```python
from build123d import *

# Parameters (mm, degrees)
SKETCH_1_W               = 40
SKETCH_1_H               = 24
EXTRUDE_1_DEPTH          = 20
EXTRUDE_2_DEPTH          = 1
EXTRUDE_2_2_DEPTH        = 1
EXTRUDE_2_3_DEPTH        = 1
EXTRUDE_2_4_DEPTH        = 1
SKETCH_1_6_W             = 1
SKETCH_1_6_H             = 24
EXTRUDE_4_DEPTH          = 20
SKETCH_2_R               = 4
EXTRUDE_5_DEPTH          = 2
FILLET_1_R               = 2
CHAMFER_1_SIZE           = 1
CHAMFER_2_SIZE           = 1
SKETCH_3_R               = 1
EXTRUDE_6_DEPTH          = 5
MIRROR_4_COPY_1_SKETCH_R = 1
MIRROR_4_COPY_1_DEPTH    = 5
MIRROR_4_COPY_2_SKETCH_R = 1
MIRROR_4_COPY_2_DEPTH    = 5


with BuildPart() as part:
    # Sketch 1 → Extrude 1 (new body)
    with BuildSketch(Plane(origin=(0, 0, 0), x_dir=(1, 0, 0), z_dir=(0, 1, 0))):
        Rectangle(SKETCH_1_W, SKETCH_1_H)
    extrude(amount=EXTRUDE_1_DEPTH)



with BuildPart() as body_2:
    # Sketch 1_4 → Extrude 2 (new body)
    with BuildSketch(Plane(origin=(0, 0, 0), x_dir=(1, 0, 0), z_dir=(0, 1, 0))):
        with BuildLine():
            Line((-21, 0), (-21, 9))
            Line((-21, 9), (-29, 6))
            Line((-29, 6), (-29, 2.5))
            Line((-29, 2.5), (-23, 2))
            ThreePointArc((-23, 2), (-21.585786438, 1.414213562), (-21, 0))
        make_face()
    extrude(amount=EXTRUDE_2_DEPTH)


with BuildPart() as body_3:
    # Sketch 1_4 → Extrude 2 2 (new body)
    with BuildSketch(Plane(origin=(0, 0, 0), x_dir=(1, 0, 0), z_dir=(0, 1, 0))):
        with BuildLine():
            Line((-29, -6), (-21, -9))
            Line((-21, -9), (-21, 0))
            ThreePointArc((-21, 0), (-21.585786438, -1.414213562), (-23, -2))
            Line((-23, -2), (-29, -2.5))
            Line((-29, -2.5), (-29, -6))
        make_face()
    extrude(amount=EXTRUDE_2_2_DEPTH)


with BuildPart() as body_4:
    # Sketch 1_4 → Extrude 2 3 (new body)
    with BuildSketch(Plane(origin=(0, 0, 0), x_dir=(1, 0, 0), z_dir=(0, 1, 0))):
        with BuildLine():
            Line((29, 6), (21, 9))
            Line((21, 9), (21, 2.5))
            Line((21, 2.5), (21, 0))
            ThreePointArc((21, 0), (21.585786438, 1.414213562), (23, 2))
            Line((23, 2), (29, 2.5))
            Line((29, 2.5), (29, 6))
        make_face()
    extrude(amount=EXTRUDE_2_3_DEPTH)


with BuildPart() as body_5:
    # Sketch 1_4 → Extrude 2 4 (new body)
    with BuildSketch(Plane(origin=(0, 0, 0), x_dir=(1, 0, 0), z_dir=(0, 1, 0))):
        with BuildLine():
            Line((21, -2.5), (21, -9))
            Line((21, -9), (29, -6))
            Line((29, -6), (29, -2.5))
            Line((29, -2.5), (23, -2))
            ThreePointArc((23, -2), (21.585786438, -1.414213562), (21, 0))
            Line((21, 0), (21, -2.5))
        make_face()
    extrude(amount=EXTRUDE_2_4_DEPTH)


with BuildPart() as part_1:
    add(part.part)

    add(body_2.part)  # Extrude 4 merges body 2

    add(body_3.part)  # Extrude 4 merges body 3

    add(body_4.part)  # Extrude 4 merges body 4

    add(body_5.part)  # Extrude 4 merges body 5
    # Sketch 1_6 → Extrude 4 (add)
    with BuildSketch(Plane(origin=(0, 0, 0), x_dir=(1, 0, 0), z_dir=(0, 1, 0))):
        with Locations((-20.5, 0)):
            Rectangle(SKETCH_1_6_W, SKETCH_1_6_H)
        Polygon((21, 12), (20, 12), (20, -12), (21, -12), (21, -9), (21, -2.5), (21, 0), (21, 2.5), (21, 9), align=None)
    extrude(amount=EXTRUDE_4_DEPTH)

    # Sketch 2 → Extrude 5 (add)
    with BuildSketch(Plane.ZY.offset(21)):
        with Locations((-6, 6)):
            Circle(SKETCH_2_R)
        with Locations(Location((6, 6, 0), (0, 0, 180))):
            Circle(SKETCH_2_R)
    extrude_5 = extrude(amount=EXTRUDE_5_DEPTH)

    # Mirror 1: Extrude 5 across plane
    add(extrude_5.mirror(Plane(origin=(0, 0, 0), x_dir=(0, 0, 1), z_dir=(1, 0, 0))))

    # Fillet 1
    fillet_1_edges = [part_1.edges().sort_by_distance(p)[0] for p in [
        (0, 20, 12),
        (0, 20, -12),
    ]]
    fillet(fillet_1_edges, radius=FILLET_1_R)

    # Chamfer 1
    chamfer_1_edges = [part_1.edges().sort_by_distance(p)[0] for p in [
        (21, 9, -12),
        (21, 20, 0),
        (21, 9, 12),
        (21, 19.414213562, 11.414213562),
        (21, 19.414213562, -11.414213562),
    ]]
    chamfer(chamfer_1_edges, length=CHAMFER_1_SIZE)

    # Chamfer 2
    chamfer_2_edges = [part_1.edges().sort_by_distance(p)[0] for p in [
        (-21, 9, -12),
        (-21, 20, 0),
        (-21, 9, 12),
        (-21, 19.414213562, 11.414213562),
        (-21, 19.414213562, -11.414213562),
    ]]
    chamfer(chamfer_2_edges, length=CHAMFER_2_SIZE)

    # Sketch 3 → Extrude 6 (add)
    with BuildSketch(Plane.ZY.offset(23)):
        with Locations((6, 6)):
            Circle(SKETCH_3_R)
    extrude_6 = extrude(amount=EXTRUDE_6_DEPTH)

    # Mirror 2: Extrude 6 across plane
    add(extrude_6.mirror(Plane.XY))

    # Mirror 3: Extrude 6 across plane
    add(extrude_6.mirror(Plane(origin=(0, 0, 0), x_dir=(0, 0, 1), z_dir=(1, 0, 0))))

    # Mirror 4 copy 1 sketch → Mirror 4 copy 1 (add)
    with BuildSketch(Plane(origin=(23, 0, 0), x_dir=(0, 0, -1), z_dir=(1, 0, 0))):
        with Locations((6, 6)):
            Circle(MIRROR_4_COPY_1_SKETCH_R)
    extrude(amount=MIRROR_4_COPY_1_DEPTH)

    # Mirror 4 copy 2 sketch → Mirror 4 copy 2 (add)
    with BuildSketch(Plane(origin=(23, 0, 0), x_dir=(0, 0, 1), z_dir=(1, 0, 0))):
        with Locations((6, -6)):
            Circle(MIRROR_4_COPY_2_SKETCH_R)
    extrude(amount=MIRROR_4_COPY_2_DEPTH)


solid = part_1.part
```
Check sheet for the modelled part. Datum: model origin and axes. Units: mm. A direction names the side the tool comes from. Round coordinates to 2 decimals unless told otherwise and drop trailing zeros. Write each loop counter-clockwise with the first axis right and the second up, starting at its lowest first coordinate (ties: lowest second). Pieces come first, ordered by that corner, then holes. Notation, with made-up numbers: (-34.5, 40.25) -> (24.5, 40.25) arc R34 ccw to (24.5, 70.25) -> close; hole circle Ø8 at (-25, 36). An arc over 180 degrees is marked (long way). One line per question, with ' | ' between items. Start each with the question number.
1. Depth check by flat-ended pin: pin 1 (9 mm diameter, centred on x = 24, z = -2.5, fed in from +Y); pin 2 (6 mm diameter, centred on y = 17, z = -5.5, fed in from -X); pin 3 (6.5 mm diameter, centred on y = 6, z = -6.5, fed in from +X); pin 4 (4 mm diameter, centred on x = -26.5, z = 5, fed in from +Y). Enter the tip coordinate at first touch or a pass-through.
2. Sectioned sample at B-B, the plane z = 1. Record the cut outline in (x, y).
3. Release check for a two-part mould opening along Y. For faces 1 (the face through (-24, 1, 4)), 2 (the face through (21.986, 9.905, 6.867)), 3 (the face through (-20.6, 18.98, -11)), 4 (the face through (-24.944, 0.493, -7.521)) record: +Y half, -Y half, draft (parallel to the pull), parting line (faces both ways), or undercut.
4. Sectioned sample at A-A, the plane y = 11.5. Record the cut outline in (x, z), then the cut area to 3 significant figures.
5. Set-up check for faces 5 (the face through (-24, 1, -5)), 6 (the face through (-28, 6, -6)), 7 (the face through (25.465, 6.676, -5.263)): record each of +Z, -Z, +X, -X, +Y, -Y from which the full face is reachable in a straight line by a thin tool's end or side.
6. Sectioned sample at C-C, the plane y = 3.25. Record the cut outline in (x, z).
7. Scan lines: line 1 along X through (y, z) = (8.25, -4.5); line 2 along X through (y, z) = (15, -3.75); line 3 along Y through (x, z) = (-24.5, -7.5). Record each from-to range of solid material in increasing order. Write a range as from..to.
Taken from the geometry:
1) pin 1: stops at y = 20 | pin 2: stops at x = -21 | pin 3: stops at x = 28 | pin 4: stops at y = 7
2) outline: (-21.27, 0) -> (21.27, 0) -> (21.27, 1) -> (21, 1) -> (21, 19) -> (20, 20) -> (-20, 20) -> (-21, 19) -> (-21, 1) -> (-21.27, 1) -> close
3) face 1: undercut | face 2: undercut | face 3: +Y half | face 4: draft
4) outline: (-21, -11) -> (-20, -12) -> (20, -12) -> (21, -11) -> (21, 11) -> (20, 12) -> (-20, 12) -> (-21, 11) -> close | area: 1,010 mm^2
5) face 5: +Z, -Z, -X | face 6: +Z, -Z, -X, +Y | face 7: +X
6) outline: (-23, -8.9) -> (-21, -8.9) -> (-21, -11) -> (-20, -12) -> (20, -12) -> (21, -11) -> (21, -8.9) -> (23, -8.9) -> (23, -3.1) -> (21, -3.1) -> (21, 3.1) -> (23, 3.1) -> (23, 8.9) -> (21, 8.9) -> (21, 11) -> (20, 12) -> (-20, 12) -> (-21, 11) -> (-21, 8.9) -> (-23, 8.9) -> (-23, 3.1) -> (-21, 3.1) -> (-21, -3.1) -> (-23, -3.1) -> close
7) line 1: x = -23..23 | line 2: x = -21..21 | line 3: y = 0..1
